from build123d import *

# Parameters (mm, degrees)
SKETCH1_R                            = 5
BOSS_EXTRUDE1_DEPTH                  = 5
BOSS_EXTRUDE3_DEPTH                  = 7.5
CUT_EXTRUDE3_DEPTH                   = 7.5
CUT_EXTRUDE3_DEPTH_BACK              = 7.5
F_95_0_03937008_DIAMETER_HOLE1_D     = 1.000000032
F_95_0_03937008_DIAMETER_HOLE1_DEPTH = 2.5
F_94_0_03937008_DIAMETER_HOLE1_D     = 1.000000032


with BuildPart() as part:
    # Sketch1 → Boss-Extrude1 (new body)
    with BuildSketch(Plane(origin=(0, 0, 0), x_dir=(1, 0, 0), z_dir=(0, 1, 0))):
        with Locations(Location((0, 0, 0), (0, 0, 270))):
            Circle(SKETCH1_R)
    extrude(amount=-BOSS_EXTRUDE1_DEPTH)

    # Sketch2 → Boss-Extrude3 (add)
    with BuildSketch(Plane.XZ.offset(5)):
        with BuildLine():
            Line((-2.5, 4.330127019), (-2.5, -4.330127019))
            ThreePointArc((-2.5, -4.330127019), (-5, 0), (-2.5, 4.330127019))
        make_face()
        with BuildLine():
            Line((2.5, 4.330127019), (2.5, -4.330127019))
            ThreePointArc((2.5, -4.330127019), (5, 0), (2.5, 4.330127019))
        make_face()
    extrude(amount=BOSS_EXTRUDE3_DEPTH)

    # Sketch3 → Cut-Extrude3 (cut, two sides: drawn at the far end of the back side and taken through both)
    with BuildSketch(Plane(origin=(-2.5, 0, 0), x_dir=(0, 0, -1), z_dir=(1, 0, 0)).offset(-CUT_EXTRUDE3_DEPTH_BACK)):
        with BuildLine():
            Line((4.330127019, -8.16987298), (5.6827841, -8.16987298))
            Line((5.6827841, -8.16987298), (5.6827841, -17.335433659))
            Line((5.6827841, -17.335433659), (-5.198770312, -17.335433659))
            Line((-5.198770312, -17.335433659), (-5.198770312, -8.16987298))
            Line((-5.198770312, -8.16987298), (-4.330127019, -8.16987298))
            ThreePointArc((-4.330127019, -8.16987298), (-3.061862179, -11.231735159), (0, -12.5))
            ThreePointArc((0, -12.5), (3.061862179, -11.231735159), (4.330127019, -8.16987298))
        make_face()
    extrude(amount=CUT_EXTRUDE3_DEPTH + CUT_EXTRUDE3_DEPTH_BACK, mode=Mode.SUBTRACT)

    # #95 (0.03937008) Diameter Hole1
    with Locations(Plane(origin=(2.5, -10, 0), x_dir=(0, 0, -1), z_dir=(-1, 0, 0))):
        with Locations((0, 0)):
            Hole(F_95_0_03937008_DIAMETER_HOLE1_D / 2, depth=F_95_0_03937008_DIAMETER_HOLE1_DEPTH)

    # #94 (0.03937008) Diameter Hole1 (through all)
    with Locations(Plane(origin=(2.5, -10, 0), x_dir=(0, 0, 1), z_dir=(1, 0, 0))):
        with Locations((0, 0)):
            Hole(F_94_0_03937008_DIAMETER_HOLE1_D / 2)

    # Sketch7 → Revolve1 (revolve)
    with BuildSketch(Plane.XY):
        with BuildLine():
            Line((0, 0), (0, 5))
            ThreePointArc((0, 5), (-3.535533906, 3.535533906), (-5, 0))
            Line((-5, 0), (0, 0))
        make_face()
    revolve(axis=Axis((0, 0, 0), (0, 1, 0)))


solid = part.part
Could you check a few things on this model? Use its own coordinates, in mm. A direction names the side the tool comes from. Coordinates: 2 decimals unless noted, no trailing zeros. Loops run counter-clockwise (first coordinate to the right, second up) from the corner with the lowest first, then second, coordinate; pieces in that order, holes last. Notation, with made-up numbers: (-24.5, -2) -> (26.5, -2) arc R23 cw to (26.5, 29) -> close; hole circle Ø3 at (10.5, 44). An arc over 180 degrees is marked (long way). Answer in a Markdown table with one row per item.
(1) For faces 3 (the face through (3.768, -9.512, -0.108)), 4 (the face through (0, -5, 0)), which set-ups out of +Z, -Z, +X, -X, +Y, -Y let a thin tool reach every point of the face, with its end or its side?
Results found:
| item | result |
|---|---|
| face 3 | +X, -X |
| face 4 | +Z, -Z, -Y |
(2) Will these pins go through, and if not, where does the flat tip stop? pin 1 Ø1.5 at (y, z) = (-7.5, 1) entering from -X; pin 2 Ø1 at (x, z) = (-1, 0) entering from +Y; pin 3 Ø4 at (x, z) = (-1, -2) entering from -Y.
Results found:
| item | result |
|---|---|
| pin 1 | stops at x = -4.99 |
| pin 2 | stops at y = 4.97 |
| pin 3 | stops at y = -12.45 |
(3) Imagine slicing it at C-C (z = -3). List the corners of the cut face in (x, y) for me, plus the area to 3 significant figures.
Results found:
| item | result |
|---|---|
| outline | (-4, -11.29) -> (-2.5, -11.29) -> (-2.5, -5) -> (2.5, -5) -> (2.5, -11.29) -> (4, -11.29) -> (4, 0) arc R4 ccw to (-4, 0) -> close |
| area | 84.0 mm^2 |
(4) Thinking about a two-plate mould opening in X: for faces 1 (the face through (-2.5, -9, 0)), 2 (the face through (-3.767, -9.512, 0.108)), which applies, released by +X, released by -X, zero draft, split by the parting line, or undercut?
Results found:
| item | result |
|---|---|
| face 1 | undercut |
| face 2 | zero draft |
(5) If I drill on probe 1 along X at (y, z) = (-7.25, 2.5); probe 2 along Z at (x, y) = (3.2, -10); probe 3 along X at (y, z) = (-6, 3.5), over which ranges is the centre line in solid material (lowest first)?
Results found:
| item | result |
|---|---|
| probe 1 | x = -4.33 to -2.5, 2.5 to 4.33 |
| probe 2 | z = -3.84 to -0.5, 0.5 to 3.84 |
| probe 3 | x = -3.57 to -2.5, 2.5 to 3.57 |
(6) Imagine slicing it at B-B (y = -5.5). List the corners of the cut face in (x, z) for me, plus the area to 3 significant figures.
Results found:
| item | result |
|---|---|
| outline | (-2.5, -4.33) -> (-2.5, 4.33) arc R5 ccw to start; (2.5, -4.33) arc R5 ccw to (2.5, 4.33) -> close |
| area | 30.7 mm^2 |
(7) Imagine slicing it at D-D (y = -10). List the corners of the cut face in (x, z) for me, plus the area to 3 significant figures.
Results found:
| item | result |
|---|---|
| outline | (-4.97, -0.5) arc R5 ccw to (-3.1, -3.92) -> (-2.5, -3.92) -> (-2.5, -0.5) -> close; (-4.97, 0.5) -> (-2.5, 0.5) -> (-2.5, 3.92) -> (-3.1, 3.92) arc R5 ccw to start; (2.5, -3.92) -> (3.1, -3.92) arc R5 ccw to (4.97, -0.5) -> (2.5, -0.5) -> close; (2.5, 0.5) -> (4.97, 0.5) arc R5 ccw to (3.1, 3.92) -> (2.5, 3.92) -> close |
| area | 25.2 mm^2 |
(8) Imagine slicing it at A-A (x = 2.75). List the corners of the cut face in (y, z) for me.
Results found:
| item | result |
|---|---|
| outline | (-9.32, -4.18) -> (0, -4.18) arc R4.18 ccw to (0, 4.18) -> (-9.32, 4.18) arc R4.33 ccw to start; hole circle Ø1 at (-10, 0) |
